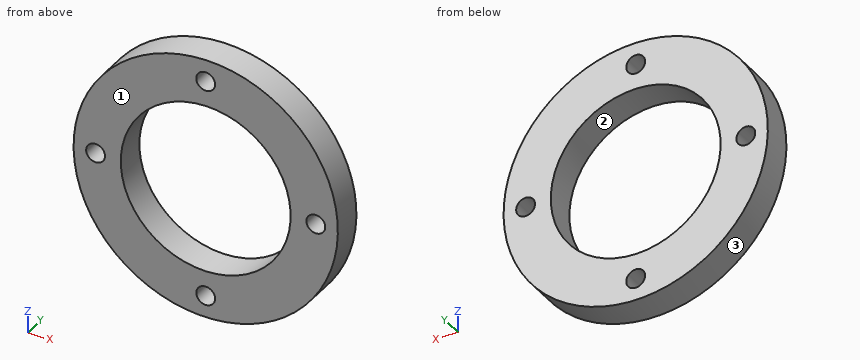
from build123d import *

# Parameters (mm, degrees)
SKETCH_1_R      = 21
SKETCH_1_R_2    = 13.5
SKETCH_1_R_3    = 1.5
EXTRUDE_1_DEPTH = 2.5


with BuildPart() as part:
    # 草图1 → 凸台-拉伸1 (new, symmetric)
    with BuildSketch(Plane(origin=(0, 0, 0), x_dir=(1, 0, 0), z_dir=(0, 1, 0))):
        with Locations(Location((0, 0, 0), (0, 0, 270))):
            Circle(SKETCH_1_R)
        with Locations(Location((0, 0, 0), (0, 0, 270))):
            Circle(SKETCH_1_R_2, mode=Mode.SUBTRACT)
        with Locations(Location((0, 17.5, 0), (0, 0, 270))):
            Circle(SKETCH_1_R_3, mode=Mode.SUBTRACT)
        with Locations(Location((17.5, 0, 0), (0, 0, 270))):
            Circle(SKETCH_1_R_3, mode=Mode.SUBTRACT)
        with Locations(Location((0, -17.5, 0), (0, 0, 270))):
            Circle(SKETCH_1_R_3, mode=Mode.SUBTRACT)
        with Locations(Location((-17.5, 0, 0), (0, 0, 270))):
            Circle(SKETCH_1_R_3, mode=Mode.SUBTRACT)
    extrude(amount=EXTRUDE_1_DEPTH, both=True)


solid = part.part
Check sheet for the modelled part. Datum: model origin and axes. Units: mm. Face numbers are marked on the shaded views. Coordinates: 2 decimals unless noted, no trailing zeros. Loops run counter-clockwise (first coordinate to the right, second up) from the corner with the lowest first, then second, coordinate; pieces in that order, holes last. Notation, with made-up numbers: (-30.5, 77) -> (-14.5, 77) arc R10 ccw to (-14.5, 87) -> close; hole circle Ø3 at (66.25, -12.75). An arc over 180 degrees is marked (long way). Answer in a Markdown table with one row per item.
1. Sectioned sample at D-D, the plane z = 17.5. Record the boundary of the cut face in (x, y).
Check values:
| item | result |
|---|---|
| outline | (-11.61, -2.5) -> (-1.5, -2.5) -> (-1.5, 2.5) -> (-11.61, 2.5) -> close; (1.5, -2.5) -> (11.61, -2.5) -> (11.61, 2.5) -> (1.5, 2.5) -> close |
2. Sectioned sample at A-A, the plane z = 0. Record the boundary of the cut face in (x, y), then the cut area to 3 significant figures.
Check values:
| item | result |
|---|---|
| outline | (-21, -2.5) -> (-19, -2.5) -> (-19, 2.5) -> (-21, 2.5) -> close; (-16, -2.5) -> (-13.5, -2.5) -> (-13.5, 2.5) -> (-16, 2.5) -> close; (13.5, -2.5) -> (16, -2.5) -> (16, 2.5) -> (13.5, 2.5) -> close; (19, -2.5) -> (21, -2.5) -> (21, 2.5) -> (19, 2.5) -> close |
| area | 45.0 mm2 |
3. Material ranges on line 1 along X through (y, z) = (0.05, 0); line 2 along Z through (x, y) = (10, 0.75); line 3 along X through (y, z) = (1.4, 3), recorded low to high. Write a range as [from, to].
Check values:
| item | result |
|---|---|
| line 1 | x = [-21, -19], [-16, -13.5], [13.5, 16], [19, 21] |
| line 2 | z = [-18.47, -9.07], [9.07, 18.47] |
| line 3 | x = [-20.78, -13.16], [13.16, 20.78] |
4. Release check for a two-part mould opening along Z. For the marked faces 1, 2 and 3 record: released by +Z, released by -Z, zero draft, split by the parting line, or undercut.
Check values:
| item | result |
|---|---|
| face 1 | zero draft |
| face 2 | undercut |
| face 3 | split by the parting line |
5. Sectioned sample at C-C, the plane x = 18. Record the boundary of the cut face in (y, z), then the cut area to 3 significant figures.
Check values:
| item | result |
|---|---|
| outline | (-2.5, -10.82) -> (2.5, -10.82) -> (2.5, -1.41) -> (-2.5, -1.41) -> close; (-2.5, 1.41) -> (2.5, 1.41) -> (2.5, 10.82) -> (-2.5, 10.82) -> close |
| area | 94.0 mm2 |
6. Sectioned sample at B-B, the plane y = -0.7. Record the boundary of the cut face in (x, z), then the cut area to 3 significant figures.
Check values:
| item | result |
|---|---|
| outline | circle Ø42 at (0, 0); hole circle Ø3 at (-17.5, 0); hole circle Ø27 at (0, 0); hole circle Ø3 at (0, -17.5); hole circle Ø3 at (0, 17.5); hole circle Ø3 at (17.5, 0) |
| area | 785 mm2 |
7. Go/stop test with a flat-tipped pin: pin 1 (1 mm diameter, centred on y = -1.5, z = 7, fed in from -X). Record where the tip stops, or that it passes through.
Check values:
| item | result |
|---|---|
| pin 1 | stops at x = -19.97 |
